from build123d import *

# Parameters (mm, degrees)
SKETCH_1_R      = 2.5
EXTRUDE_1_DEPTH = 4
SKETCH_2_W      = 6
SKETCH_2_H      = 8
SKETCH_2_R      = 2.5
EXTRUDE_2_DEPTH = 5
CHAMFER_1_SIZE  = 1
FILLET_1_R      = 1


with BuildPart() as part:
    # 草图1 → 凸台-拉伸1 (new body)
    with BuildSketch(Plane.XY):
        with BuildLine():
            Line((5, 10), (5, -10))
            ThreePointArc((5, -10), (0, -15), (-5, -10))
            Line((-5, -10), (-5, 10))
            ThreePointArc((-5, 10), (0, 15), (5, 10))
        make_face()
        with Locations((0, 10)):
            Circle(SKETCH_1_R, mode=Mode.SUBTRACT)
        with Locations((0, -10)):
            Circle(SKETCH_1_R, mode=Mode.SUBTRACT)
    extrude(amount=EXTRUDE_1_DEPTH)

    # 草图2 → 凸台-拉伸2 (add)
    with BuildSketch(Plane(origin=(5, 0, 0), x_dir=(0, 0, -1), z_dir=(1, 0, 0))):
        with Locations((-1, 0)):
            Rectangle(SKETCH_2_W, SKETCH_2_H)
        with Locations(Location((-0.9, 0, 0), (0, 0, 68.899803976))):
            Circle(SKETCH_2_R, mode=Mode.SUBTRACT)
    extrude(amount=EXTRUDE_2_DEPTH)

    # 倒角1
    chamfer_1_edges = [part.edges().sort_by_distance(p)[0] for p in [
        (5, -4, 2),
        (5, 4, 2),
    ]]
    chamfer(chamfer_1_edges, length=CHAMFER_1_SIZE)

    # 圆角1
    # the kernel refuses this fillet: 1 mm, written as the material it takes off along each edge
    with BuildSketch(Plane(origin=(5, 6.5, -2), x_dir=(0, 0, 1), z_dir=(0, -1, 0))) as fillet_1_piece_1:
        with BuildLine():
            CenterArc((FILLET_1_R, -FILLET_1_R), FILLET_1_R, 90, 90)
            Line((0, -FILLET_1_R), (0, 0))
            Line((0, 0), (FILLET_1_R, 0))
        make_face()
    extrude(amount=13, mode=Mode.SUBTRACT)
    with BuildSketch(Plane(origin=(2.5, -4, -2), x_dir=(0, 0, 1), z_dir=(1, 0, 0))) as fillet_1_piece_2:
        with BuildLine():
            CenterArc((FILLET_1_R, -FILLET_1_R), FILLET_1_R, 90, 90)
            Line((0, -FILLET_1_R), (0, 0))
            Line((0, 0), (FILLET_1_R, 0))
        make_face()
    extrude(amount=10, mode=Mode.SUBTRACT)
    with BuildSketch(Plane(origin=(2.5, 4, -2), x_dir=(0, 0, 1), z_dir=(1, 0, 0))) as fillet_1_piece_3:
        with BuildLine():
            CenterArc((FILLET_1_R, FILLET_1_R), FILLET_1_R, 180, 90)
            Line((0, FILLET_1_R), (0, 0))
            Line((0, 0), (FILLET_1_R, 0))
        make_face()
    extrude(amount=10, mode=Mode.SUBTRACT)


solid = part.part
Source: CAD feature listing. Evaluate the final solid. Frame: model axes, mm. A direction names the side the tool comes from. Round coordinates to 2 decimals unless told otherwise and drop trailing zeros. Write each loop counter-clockwise with the first axis right and the second up, starting at its lowest first coordinate (ties: lowest second). Pieces come first, ordered by that corner, then holes. Notation, with made-up numbers: M 30.5,-32.75 L 74.5,-32.75 A28 ccw 74.5,-5.75 Z; hole C -8,21 d2. An arc over 180 degrees is marked long. One line per item, written item: value. Start each with the question number.
Item 1: Pin query (flat end, axial travel): pin 1 (0.8 mm diameter, centred on y = 3, z = -0.5, fed in from -X); pin 2 (1.2 mm diameter, centred on y = -7.5, z = 2.5, fed in from +X); pin 3 (3 mm diameter, centred on x = 2, z = -1, fed in from -Y). Return the tip coordinate at first contact, or that it passes through.
Item 2: Mould query, pull axis Y, two halves, no side actions, for faces 1 (the flat face through (1, 0, 4)), 2 (the flat face through (5, 0, 1)), 3 (the cylindrical face through (7.465, -1.384, -1.182)), 4 (the flat face through (8, -4, 2)). Classes: pulls with the +Y half, pulls with the -Y half, needs draft (parallel to the pull), parting line crosses it, or undercut.
Item 3: Section query A-A (x = 0). Return the cut outline in (y, z), plus the area to 3 significant figures.
Item 4: Ray query, L1, parallel to Y at x = 0, z = 3.1; L2, parallel to Z at x = 8.2, y = 0; L3, parallel to Y at x = 7, z = 0.9. Return the intervals inside material, ascending. Write a range as from..to.
Item 5: Section query B-B (y = 0). Return the cut outline in (x, z), plus the area to 3 significant figures.
Item 6: Set-up query: faces 5 (the flat face through (5, -3.1, -0.5)), 6 (the flat face through (5, -7, 2)), 7 (the flat face through (5, 8, 2)). Return all of +Z, -Z, +X, -X, +Y, -Y with unobstructed straight access to the full face (end or side cutting, diameter ignored); none if empty.
Item 7: Section query C-C (z = 0.9). Return the cut outline in (x, y).
Item 8: Section query D-D (y = 11.25). Return the cut outline in (x, z), plus the area to 3 significant figures.
Result set:
1. pin 1: stops at x = 5
1. pin 2: stops at x = 5
1. pin 3: stops at y = -14.92
2. face 1: needs draft
2. face 2: undercut
2. face 3: undercut
2. face 4: pulls with the -Y half
3. outline: M -15,0 L -12.5,0 L -12.5,4 L -15,4 Z; M -7.5,0 L 7.5,0 L 7.5,4 L -7.5,4 Z; M 12.5,0 L 15,0 L 15,4 L 12.5,4 Z
3. area: 80.0 mm²
4. L1: y = -15..-12.5, -7.5..7.5, 12.5..15
4. L2: z = -2..-1.6, 3.4..4
4. L3: y = -4..-2.5, 2.5..4
5. outline: M -5,0 L 5,0 L 5,3.4 L 10,3.4 L 10,4 L -5,4 Z; M 5.2,-1.6 A1 ccw 6,-2 L 10,-2 L 10,-1.6 Z
5. area: 44.8 mm²
6. face 5: -Z, -X, +Y, -Y
6. face 6: +Z, -Z, +X, -Y
6. face 7: +Z, -Z, +X, +Y
7. outline: M -5,-10 A5 ccw 5,-10 L 5,-5 L 6,-4 L 10,-4 L 10,-2.5 L 5,-2.5 L 5,2.5 L 10,2.5 L 10,4 L 6,4 L 5,5 L 5,10 A5 ccw -5,10 Z; hole C 0,-10 d5; hole C 0,10 d5
8. outline: M -4.84,0 L -2.17,0 L -2.17,4 L -4.84,4 Z; M 2.17,0 L 4.84,0 L 4.84,4 L 2.17,4 Z
8. area: 21.4 mm²
